from build123d import *

# Parameters (mm, degrees)
SKETCH1_R           = 3.5
BOSS_EXTRUDE1_DEPTH = 5
SKETCH2_R           = 5
BOSS_EXTRUDE2_DEPTH = 3
CHAMFER1_SIZE       = 5
CHAMFER1_SIZE_2     = 1.5
SKETCH3_R           = 2.6
CUT_EXTRUDE1_DEPTH  = 20


with BuildPart() as part:
    # Sketch1 → Boss-Extrude1 (new body)
    with BuildSketch(Plane(origin=(0, 0, 0), x_dir=(1, 0, 0), z_dir=(0, 1, 0))):
        with Locations(Location((0, 0, 0), (0, 0, 270))):
            Circle(SKETCH1_R)
    extrude(amount=BOSS_EXTRUDE1_DEPTH)

    # Sketch2 → Boss-Extrude2 (add)
    with BuildSketch(Plane(origin=(0, 5, 0), x_dir=(1, 0, 0), z_dir=(0, 1, 0))):
        with Locations(Location((0, 0, 0), (0, 0, 270))):
            Circle(SKETCH2_R)
    extrude(amount=BOSS_EXTRUDE2_DEPTH)

    # Chamfer1
    # the kernel refuses this chamfer: 5, 1.5 mm, written as the material it takes off along each edge
    with BuildSketch(Plane(origin=(0, 8, 0), x_dir=(0, 0, 1), z_dir=(-1, 0, 0))) as chamfer1_piece_1:
        Polygon((5, -CHAMFER1_SIZE), (5 - CHAMFER1_SIZE_2, 0), (5, 0), align=None)
    revolve(axis=Axis((0, 8, 0), (0, 1, 0)), mode=Mode.SUBTRACT)

    # Sketch3 → Cut-Extrude1 (cut)
    with BuildSketch(Plane(origin=(0, 8, 0), x_dir=(1, 0, 0), z_dir=(0, 1, 0))):
        with Locations(Location((0, 0, 0), (0, 0, 270))):
            Circle(SKETCH3_R)
    extrude(amount=-CUT_EXTRUDE1_DEPTH, mode=Mode.SUBTRACT)


solid = part.part
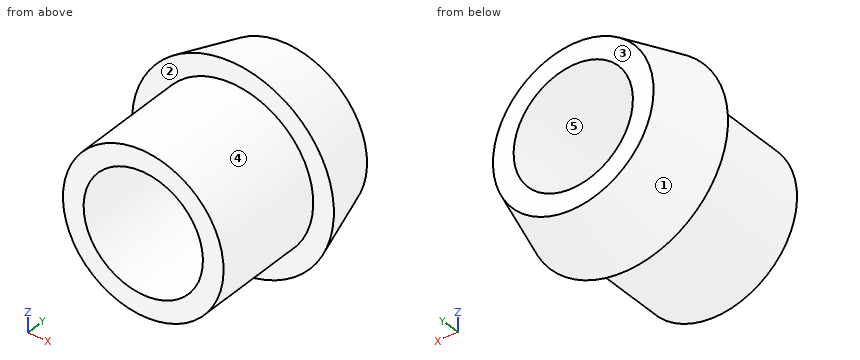
For this review, take the finished solid that the model builds, in its own axes (mm). Face numbers are marked on the shaded views. A direction names the side the tool comes from. Give positions to 0.01 mm unless a question says otherwise; leave off trailing zeros. Loops run counter-clockwise (first coordinate to the right, second up) from the corner with the lowest first, then second, coordinate; pieces in that order, holes last.
Item 1: Take a section at B-B, the plane x = 0. State the section outline as (y, z) points.
Item 2: Draft analysis for pull direction X (two halves, no side actions). For the marked faces 3, 4 and 5, state which applies: +X half, -X half, draft (parallel to the pull), parting line (faces both ways), or undercut.
Item 3: Take a section at C-C, the plane y = 4.75. State the section outline as (x, z) points.
Item 4: Insertion check: pin 1 (1.5 mm diameter, centred on y = 6, z = 2, fed in from -X); pin 2 (2.5 mm diameter, centred on x = 1, z = 0, fed in from -Y). Each pin has a flat end and moves straight along its axis. Give the tip position at first contact, or say it passes through.
Item 5: For line 1 along X through (y, z) = (3.75, 0); line 2 along Z through (x, y) = (-0.25, 4.25); line 3 along Z through (x, y) = (0.5, 7.25), list the stretches that pass through material, from the lowest coordinate up.
Item 6: Tool access review of the marked faces 1 and 2: name each direction out of +Z, -Z, +X, -X, +Y, -Y from which nothing blocks a thin tool from reaching the whole face with its end or side.
Item 7: Take a section at A-A, the plane z = 0. State the section outline as (x, y) points, and give its area (3 significant figures).
Calculated:
1. outline: (0, -3.5) - (5, -3.5) - (5, -4.4) - (8, -3.5) - (8, -2.6) - (0, -2.6) - close; (0, 2.6) - (8, 2.6) - (8, 3.5) - (5, 4.4) - (5, 3.5) - (0, 3.5) - close
2. face 3: draft
2. face 4: parting line
2. face 5: undercut
3. outline: circle Ø7 at (0, 0); hole circle Ø5.2 at (0, 0)
4. pin 1: stops at x = -4
4. pin 2: passes through
5. line 1: x = -3.5 to -2.6, 2.6 to 3.5
5. line 2: z = -3.49 to -2.59, 2.59 to 3.49
5. line 3: z = -3.69 to -2.55, 2.55 to 3.69
6. face 1: +Y
6. face 2: -Y
7. outline: (-4.4, 5) - (-3.5, 5) - (-3.5, 0) - (-2.6, 0) - (-2.6, 8) - (-3.5, 8) - close; (2.6, 0) - (3.5, 0) - (3.5, 5) - (4.4, 5) - (3.5, 8) - (2.6, 8) - close
7. area: 17.1 mm2
